Work out the finished part from the listing and answer in its coordinate system (mm). Face numbers are marked on the shaded views. A direction names the side the tool comes from. Coordinates: 2 decimals unless noted, no trailing zeros. Write each loop counter-clockwise with the first axis right and the second up, starting at its lowest first coordinate (ties: lowest second). Pieces come first, ordered by that corner, then holes. Notation, with made-up numbers: (42.5, 16.25) - (62.5, 16.25) arc R19 cw to (62.5, 25.25) - close; hole circle Ø7 at (33.5, 31.25). An arc over 180 degrees is marked (long way). One line per item, written item: value.
```python
from build123d import *


with BuildPart() as part:
    # 草图1 → 旋转1 (revolve)
    with BuildSketch(Plane.XY, mode=Mode.PRIVATE) as revolve_1_sk:
        with BuildLine():
            Line((20, 0), (30, 0))
            Line((30, 0), (30, 10))
            Line((30, 10), (20, 10))
            Line((20, 10), (20, 40))
            ThreePointArc((20, 40), (10, 43.819660113), (0, 40))
            Line((0, 40), (0, 10))
            Line((0, 10), (-10, 10))
            Line((-10, 10), (-10, 0))
            Line((-10, 0), (0, 0))
            Line((0, 0), (20, 0))
        make_face()
    revolve(revolve_1_sk.sketch.rotate(Axis((0, 0, 0), (1, 0, 0)), 90), axis=Axis((0, 0, 0), (1, 0, 0)))


solid = part.part
```
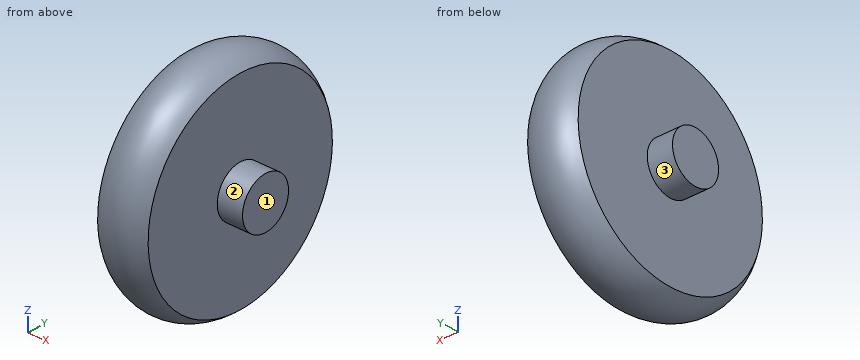
Item 1: Consider probe 1 along X at (y, z) = (-28.5, -4); probe 2 along Y at (x, z) = (-6.5, -1); probe 3 along Y at (x, z) = (6.5, -1.5). Determine where each line is inside the solid, lowest interval first.
Evaluation:
probe 1: x = 0 to 20
probe 2: y = -9.95 to 9.95
probe 3: y = -43.38 to 43.38
Item 2: Section A-A, the plane y = 0 is taken. Determine the outline of the cut face in (x, z), then the cut area to 3 significant figures.
Evaluation:
outline: (-10, -10) - (0, -10) - (0, -40) arc R15 ccw to (20, -40) - (20, -10) - (30, -10) - (30, 10) - (20, 10) - (20, 40) arc R15 ccw to (0, 40) - (0, 10) - (-10, 10) - close
area: 2,100 mm2
Item 3: Section C-C, the plane x = 27.5 is taken. Determine the outline of the cut face in (y, z).
Evaluation:
outline: circle Ø20 at (0, 0)
Item 4: Given pin 1 (1 mm diameter, centred on x = 1, z = -21, fed in from -Y); pin 2 (3 mm diameter, centred on y = 19, z = -6.5, fed in from -X); pin 3 (10 mm diameter, centred on x = 16, y = -34.5, fed in from +Z), each flat-ended and moving along its own axis, determine where each tip first touches the part or whether it passes through.
Evaluation:
pin 1: stops at y = -35.52
pin 2: stops at x = 0
pin 3: stops at z = 31.27
Item 5: Which of the six approach directions +Z, -Z, +X, -X, +Y, -Y give full straight-line access (tool end or side, diameter ignored) to the marked faces 1, 2 and 3?
Evaluation:
face 1: +Z, -Z, +X, +Y, -Y
face 2: +X
face 3: -X
